```python
from build123d import *

# Parameters (mm, degrees)
SKETCH1_R           = 25.4
SKETCH1_R_2         = 12.7
BOSS_EXTRUDE1_DEPTH = 25.4
SKETCH4_R           = 31.75
SKETCH4_R_2         = 12.7
BOSS_EXTRUDE3_DEPTH = 3.175


with BuildPart() as part:
    # Sketch1 → Boss-Extrude1 (new body)
    with BuildSketch(Plane(origin=(0, 0, 0), x_dir=(1, 0, 0), z_dir=(0, 1, 0))):
        with Locations(Location((0, 0, 0), (0, 0, 270))):
            Circle(SKETCH1_R)
        with Locations(Location((0, 0, 0), (0, 0, 270))):
            Circle(SKETCH1_R_2, mode=Mode.SUBTRACT)
    extrude(amount=BOSS_EXTRUDE1_DEPTH)

    # Sketch4 → Boss-Extrude3 (add)
    with BuildSketch(Plane(origin=(0, 25.4, 0), x_dir=(1, 0, 0), z_dir=(0, 1, 0))):
        with Locations(Location((0, 0, 0), (0, 0, 270))):
            Circle(SKETCH4_R)
        with Locations(Location((0, 0, 0), (0, 0, 270))):
            Circle(SKETCH4_R_2, mode=Mode.SUBTRACT)
    boss_extrude3 = extrude(amount=BOSS_EXTRUDE3_DEPTH)

    # Mirror2: Boss-Extrude3 across plane
    add(boss_extrude3.mirror(Plane.ZX.offset(12.7)))


solid = part.part
```
Build history of the part. All positions in model axes, mm. A direction names the side the tool comes from. Give positions to 0.01 mm unless a question says otherwise; leave off trailing zeros. Loops run counter-clockwise (first coordinate to the right, second up) from the corner with the lowest first, then second, coordinate; pieces in that order, holes last. Notation, with made-up numbers: (-25, 77) -> (27, 77) arc R27 cw to (27, 99) -> close; hole circle Ø8 at (16, 22.5). An arc over 180 degrees is marked (long way). One line per question, with ' | ' between items. Start each with the question number.
1) Cut at C-C (x = -20.5). Give the cut face in (y, z) (3 decimals).
2) Cut at D-D (y = 20). Give the cut face in (x, z).
3) Cut at B-B (z = 0). Give the cut face in (x, y) (3 decimals), plus the area to 3 significant figures.
4) Cut at A-A (x = 0). Give the cut face in (y, z) (3 decimals), plus the area to 3 significant figures.
5) Probe L1, parallel to Y at x = 27, z = 0.5 (3 decimals); L2, parallel to X at y = 19, z = 0; L3, parallel to X at y = 24, z = -10.5. List the from-to ranges inside material, lowest first.
6) Two-plate mould, pull along X, no slides. Class faces 1 (the cylindrical face through (-30.995, -1.565, -6.883)), 2 (the flat face through (21.3, 0, -14.3)), 3 (the cylindrical face through (-7.7, 12.9, -10.1)): released by +X, released by -X, zero draft, split by the parting line, or undercut.
7) Pin check, flat tips, straight feed: pin 1 (1 mm diameter, centred on y = 22, z = -9.5, fed in from +X); pin 2 (4 mm diameter, centred on y = 21.5, z = -7.5, fed in from -X); pin 3 (2 mm diameter, centred on x = -3, y = 10, fed in from +Z); pin 4 (15 mm diameter, centred on x = 0, z = 0, fed in from -Y). Stop position of each tip, or through.
8) 3-axis set-ups, long thin cutter, end or side, ignore diameter. For faces 4 (the flat face through (21.3, 25.4, -14.3)), 5 (the flat face through (-14, 28.575, 0)): which of +Z, -Z, +X, -X, +Y, -Y reach the whole face in a straight line?
Return value:
1) outline: (-3.175, -24.245) -> (0, -24.245) -> (0, -14.997) -> (25.4, -14.997) -> (25.4, -24.245) -> (28.575, -24.245) -> (28.575, 24.245) -> (25.4, 24.245) -> (25.4, 14.997) -> (0, 14.997) -> (0, 24.245) -> (-3.175, 24.245) -> close
2) outline: circle Ø50.8 at (0, 0); hole circle Ø25.4 at (0, 0)
3) outline: (-31.75, -3.175) -> (-12.7, -3.175) -> (-12.7, 28.575) -> (-31.75, 28.575) -> (-31.75, 25.4) -> (-25.4, 25.4) -> (-25.4, 0) -> (-31.75, 0) -> close; (12.7, -3.175) -> (31.75, -3.175) -> (31.75, 0) -> (25.4, 0) -> (25.4, 25.4) -> (31.75, 25.4) -> (31.75, 28.575) -> (12.7, 28.575) -> close | area: 887 mm^2
4) outline: (-3.175, -31.75) -> (0, -31.75) -> (0, -25.4) -> (25.4, -25.4) -> (25.4, -31.75) -> (28.575, -31.75) -> (28.575, -12.7) -> (-3.175, -12.7) -> close; (-3.175, 12.7) -> (28.575, 12.7) -> (28.575, 31.75) -> (25.4, 31.75) -> (25.4, 25.4) -> (0, 25.4) -> (0, 31.75) -> (-3.175, 31.75) -> close | area: 887 mm^2
5) L1: -3.175 to 0, 25.4 to 28.575 | L2: -25.4 to -12.7, 12.7 to 25.4 | L3: -23.13 to -7.14, 7.14 to 23.13
6) face 1: split by the parting line | face 2: zero draft | face 3: undercut
7) pin 1: x = 23.75 | pin 2: x = -24.8 | pin 3: z = 25.32 | pin 4: through
8) face 4: none | face 5: +Z, -Z, +X, -X, +Y
